```python
from build123d import *

# Parameters (mm, degrees)
BOSS_EXTRUDE2_DEPTH = 7
FILLET1_R           = 1
FILLET2_R           = 1


with BuildPart() as part:
    # Sketch4 → Boss-Extrude2 (new body)
    with BuildSketch(Plane(origin=(0, 0, 0), x_dir=(0, 0, -1), z_dir=(1, 0, 0))):
        with BuildLine():
            Line((-82.536856532, 31.771329741), (-81.846213718, 44.949579673))
            Line((-81.846213718, 44.949579673), (-77.851695579, 44.740235848))
            ThreePointArc((-77.851695579, 44.740235848), (-76.552846322, 43.836343889), (-76.786856532, 42.271329741))
            Line((-76.786856532, 42.271329741), (-76.786856532, 31.771329741))
            Line((-76.786856532, 31.771329741), (-72.536856532, 31.771329741))
            Line((-72.536856532, 31.771329741), (-72.536856532, 25.771329741))
            Line((-72.536856532, 25.771329741), (-87.536856532, 25.771329741))
            Line((-87.536856532, 25.771329741), (-87.536856532, 49.271329741))
            Line((-87.536856532, 49.271329741), (-77.036856532, 49.271329741))
            Line((-77.036856532, 49.271329741), (-77.036856532, 45.271329741))
            Line((-77.036856532, 45.271329741), (-82.536856532, 45.271329741))
            Line((-82.536856532, 45.271329741), (-82.536856532, 31.771329741))
        make_face()
    boss_extrude2 = extrude(amount=BOSS_EXTRUDE2_DEPTH)

    # Fillet1
    fillet1_edges = [part.edges().sort_by_distance(p)[0] for p in [
        (3.5, 44.949579673, 81.846213718),
    ]]
    fillet(fillet1_edges, radius=FILLET1_R)

    # Fillet2
    fillet2_edges = [part.edges().sort_by_distance(p)[0] for p in [
        (3.5, 45.271329741, 82.536856532),
    ]]
    fillet(fillet2_edges, radius=FILLET2_R)

    # Mirror2: Boss-Extrude2 across plane
    add(boss_extrude2.mirror(Plane(origin=(7, 31.771329741, 72.536856532), x_dir=(1, 0, 0), z_dir=(0, 0, 1))))


solid = part.part
```
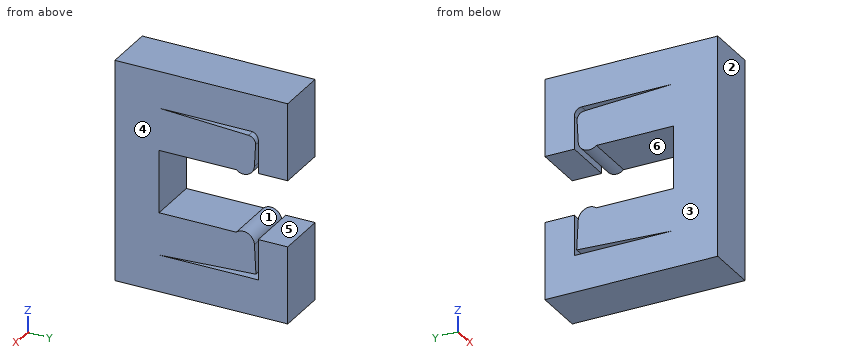
Design review of the part built by this model. Coordinates are the model's own, in mm. Face numbers are marked on the shaded views. A direction names the side the tool comes from. Round coordinates to 2 decimals unless told otherwise and drop trailing zeros. Write each loop counter-clockwise with the first axis right and the second up, starting at its lowest first coordinate (ties: lowest second). Pieces come first, ordered by that corner, then holes.
Item 1: For the marked faces 4, 5 and 6, list the 3-axis set-ups (+Z, -Z, +X, -X, +Y, -Y) from which the entire face can be reached by the end or side of a thin tool; tool diameter is ignored.
Item 2: We need section C-C on x = 2.75. Write out the cut boundary in (y, z), and give its area (3 significant figures).
Item 3: The part is to be moulded in two halves that separate along Y. For the marked faces 1, 2 and 3, say which applies: +Y half, -Y half, draft (parallel to the pull), parting line (faces both ways), or undercut.
Item 4: We need section A-A on y = 47.5. Write out the cut boundary in (x, z).
Item 5: We need section B-B on z = 64. Write out the cut boundary in (x, y), and give its area (3 significant figures).
Item 6: For probe 1 along Z at (x, y) = (5.25, 45.5); probe 2 along Z at (x, y) = (3.25, 35.5); probe 3 along Y at (x, z) = (3.25, 69.5), list the stretches that pass through material, from the lowest coordinate up.
Item 7: Clearance check with flat-ended pins moving along their axes: pin 1 Ø1.5 at (x, z) = (6, 75.5) entering from +Y; pin 2 Ø2 at (y, z) = (35, 80.5) entering from -X. State where each tip first meets the part, or that it passes through.
Item 8: We need section D-D on y = 39.25. Write out the cut boundary in (x, z), and give its area (3 significant figures).
Returned:
1. face 4: +Z, -Z, +X, +Y, -Y
1. face 5: +X, -X, +Y
1. face 6: +X, -X
2. outline: (25.77, 57.54) - (49.27, 57.54) - (49.27, 68.04) - (45.27, 68.04) - (45.27, 62.54) - (31.77, 62.54) - (44.95, 63.23) - (44.74, 67.22) arc R1.5 ccw to (42.27, 68.29) - (31.77, 68.29) - (31.77, 76.79) - (42.27, 76.79) arc R1.5 ccw to (44.74, 77.85) - (44.9, 80.85) arc R1 ccw to (43.95, 81.9) - (31.77, 82.54) - (44.27, 82.54) arc R1 cw to (45.27, 81.54) - (45.27, 77.04) - (49.27, 77.04) - (49.27, 87.54) - (25.77, 87.54) - close
2. area: 541 mm2
3. face 1: undercut
3. face 2: -Y half
3. face 3: draft
4. outline: (0, 57.54) - (7, 57.54) - (7, 68.04) - (0, 68.04) - close; (0, 77.04) - (7, 77.04) - (7, 87.54) - (0, 87.54) - close
5. outline: (0, 25.77) - (7, 25.77) - (7, 44.91) - (0, 44.91) - close; (0, 45.27) - (7, 45.27) - (7, 49.27) - (0, 49.27) - close
5. area: 162 mm2
6. probe 1: z = 57.54 to 68.04, 77.04 to 87.54
6. probe 2: z = 57.54 to 62.54, 62.73 to 68.29, 76.79 to 82.34, 82.54 to 87.54
6. probe 3: y = 25.77 to 31.77
7. pin 1: stops at y = 31.77
7. pin 2: stops at x = 0
8. outline: (0, 57.54) - (7, 57.54) - (7, 62.54) - (0, 62.54) - close; (0, 62.93) - (7, 62.93) - (7, 68.29) - (0, 68.29) - close; (0, 76.79) - (7, 76.79) - (7, 82.14) - (0, 82.14) - close; (0, 82.54) - (7, 82.54) - (7, 87.54) - (0, 87.54) - close
8. area: 145 mm2
